```python
from build123d import *

# Parameters (mm, degrees)
CROQUIS1_R              = 32.5
SALIENTE_EXTRUIR1_DEPTH = 70
CROQUIS2_R              = 1.5
CORTAR_EXTRUIR1_DEPTH   = 5
CROQUIS2_3_R            = 26.5
CROQUIS2_3_R_2          = 20
CORTAR_EXTRUIR2_DEPTH   = 7.4


with BuildPart() as part:
    # Croquis1 → Saliente-Extruir1 (new body)
    with BuildSketch(Plane(origin=(0, 0, 0), x_dir=(1, 0, 0), z_dir=(0, 1, 0))):
        Circle(CROQUIS1_R)
    extrude(amount=SALIENTE_EXTRUIR1_DEPTH)

    # Croquis2 → Cortar-Extruir1 (cut)
    with BuildSketch(Plane(origin=(0, 70, 0), x_dir=(1, 0, 0), z_dir=(0, 1, 0))):
        with Locations((15, 0)):
            Circle(CROQUIS2_R)
        with Locations((7.5, -12.990381057)):
            Circle(CROQUIS2_R)
        with Locations((-7.5, -12.990381057)):
            Circle(CROQUIS2_R)
        with Locations((-15, 0)):
            Circle(CROQUIS2_R)
        with Locations((-7.5, 12.990381057)):
            Circle(CROQUIS2_R)
        with Locations((7.5, 12.990381057)):
            Circle(CROQUIS2_R)
    extrude(amount=-CORTAR_EXTRUIR1_DEPTH, mode=Mode.SUBTRACT)

    # Croquis2<3> → Cortar-Extruir2 (cut)
    with BuildSketch(Plane(origin=(0, 70, 0), x_dir=(1, 0, 0), z_dir=(0, 1, 0))):
        Circle(CROQUIS2_3_R)
        Circle(CROQUIS2_3_R_2, mode=Mode.SUBTRACT)
    extrude(amount=-CORTAR_EXTRUIR2_DEPTH, mode=Mode.SUBTRACT)


solid = part.part
```
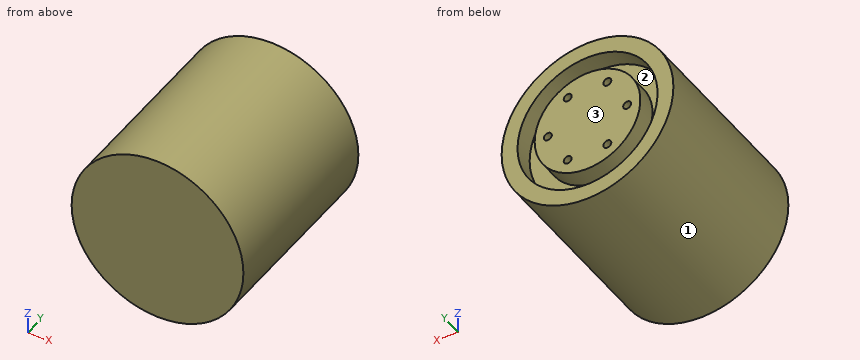
Input: part model. Units: mm. Frame: model coordinates. Face numbers are marked on the shaded views. Give positions to 0.01 mm unless a question says otherwise; leave off trailing zeros. Order: outer loops, then holes, each group sorted by start corner. A loop starts at its lowest first (then second) coordinate and runs counter-clockwise, first axis right, second up. Notation, with made-up numbers: (73, 39.25) - (129, 39.25) arc R16 ccw to (129, 44.25) - close; hole circle Ø10 at (-8, -16.75). An arc over 180 degrees is marked (long way). One line per item, written item: value.
1. Line query: probe 1 along X at (y, z) = (68, 0); probe 2 along Z at (x, y) = (0, 68); probe 3 along X at (y, z) = (64, -18). Output: solid intervals per line, ascending.
Determined:
probe 1: -32.5 to -26.5, -20 to -16.5, -13.5 to 13.5, 16.5 to 20, 26.5 to 32.5
probe 2: -32.5 to -26.5, -20 to 20, 26.5 to 32.5
probe 3: -27.06 to -19.45, -8.72 to 8.72, 19.45 to 27.06
2. Pin query (flat end, axial travel): pin 1 Ø2.5 at (x, z) = (-7.5, -12.99) entering from +Y; pin 2 Ø2 at (y, z) = (22, -15) entering from +X; pin 3 Ø5 at (y, z) = (42, -24) entering from -X. Return the tip coordinate at first contact, or that it passes through.
Determined:
pin 1: y = 65
pin 2: x = 29.33
pin 3: x = -24.37
3. Cut plane B-B, the plane z = 0. Output: boundary loops of the cut face in (x, y), and give its area (3 significant figures).
Determined:
outline: (-32.5, 0) - (32.5, 0) - (32.5, 70) - (26.5, 70) - (26.5, 62.6) - (20, 62.6) - (20, 70) - (16.5, 70) - (16.5, 65) - (13.5, 65) - (13.5, 70) - (-13.5, 70) - (-13.5, 65) - (-16.5, 65) - (-16.5, 70) - (-20, 70) - (-20, 62.6) - (-26.5, 62.6) - (-26.5, 70) - (-32.5, 70) - close
area: 4,420 mm2
4. Cut plane A-A, the plane x = 0. Output: boundary loops of the cut face in (y, z), and give its area (3 significant figures).
Determined:
outline: (0, -32.5) - (70, -32.5) - (70, -26.5) - (62.6, -26.5) - (62.6, -20) - (70, -20) - (70, 20) - (62.6, 20) - (62.6, 26.5) - (70, 26.5) - (70, 32.5) - (0, 32.5) - close
area: 4,450 mm2
5. Cut plane D-D, the plane z = 21. Output: boundary loops of the cut face in (x, y).
Determined:
outline: (-24.8, 0) - (24.8, 0) - (24.8, 70) - (16.16, 70) - (16.16, 62.6) - (-16.16, 62.6) - (-16.16, 70) - (-24.8, 70) - close
6. Cut plane C-C, the plane y = 60. Output: boundary loops of the cut face in (x, z).
Determined:
outline: circle Ø65 at (0, 0)
7. Draft query along Z for the marked faces 1, 2 and 3. Return one class per face: released by +Z, released by -Z, zero draft, split by the parting line, or undercut.
Determined:
face 1: split by the parting line
face 2: undercut
face 3: zero draft
